For this review, take the finished solid that the model builds, in its own axes (mm). Face numbers are marked on the shaded views. A direction names the side the tool comes from. Round coordinates to 2 decimals unless told otherwise and drop trailing zeros. Order: outer loops, then holes, each group sorted by start corner. A loop starts at its lowest first (then second) coordinate and runs counter-clockwise, first axis right, second up. Notation, with made-up numbers: (26.5, -16) -> (36.5, -16) arc R21 ccw to (36.5, -11) -> close; hole circle Ø11 at (8.25, 58.5). An arc over 180 degrees is marked (long way). Answer in a Markdown table with one row per item.
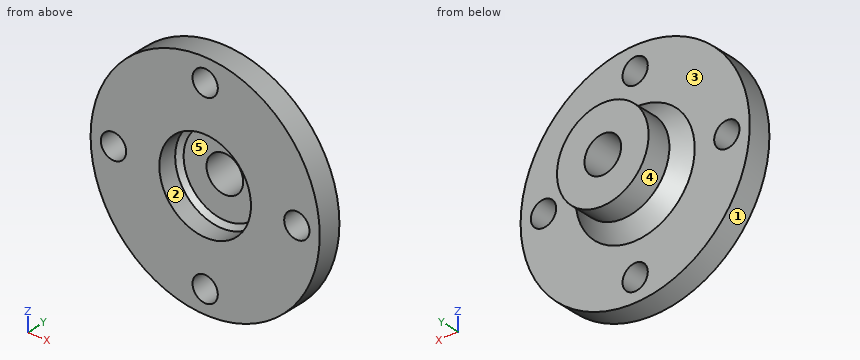
Autodesk Inventor part; units mm, degrees
ref_plane "Work Plane3" through (0, 8.5344, 0) normal (1, 0, 0) x (0, 1, 0)
ref_plane "YZ Plane" through (0, 0, 0) normal (1, 0, 0) x (0, 1, 0)
ref_plane "XZ Plane" through (0, 0, 0) normal (0, 1, 0) x (-1, 0, 0)
sketch "Sketch1" plane through (0, 0, 0) normal (0, 1, 0) x (-1, 0, 0)
  circle A0 centre (0, 0) radius 15.875
  circle A1 centre (0, 0) radius 6.35
  circle A2 centre (0, 12.7) radius 1.75
  circle A3 centre (-12.7, 0) radius 1.75
  circle A4 centre (0, -12.7) radius 1.75
  circle A5 centre (12.7, 0) radius 1.75
  dimension "d1" = 12.7
  dimension "d6" = 3.5
  dimension "d7" = 3.5
  dimension "d8" = 3.5
  dimension "d9" = 3.5
extrude "Extrusion1" add sketch "Sketch1" along normal blind 3.2258
sketch "Sketch2" plane through (0, 3.2258, 0) normal (0, 1, 0) x (1, 0, 0)
  circle A0 centre (0, 0) radius 6.35
  circle A1 centre (0, 0) radius 2.54
  dimension "d12" = 5.08
extrude "Extrusion2" add sketch "Sketch2" along normal blind 5.3086
sketch "Sketch3" plane through (0, 8.5344, 0) normal (0, 1, 0) x (1, 0, 0)
  line L0 (0, 0) -> (6.35, 0)
  circle A0 centre (0, 0) radius 6.35
  line L1 (0, 0) -> (-6.35, 0)
ref_plane "Work Plane3" through (0, 8.5344, 0) normal (1, 0, 0) x (0, 1, 0)
sketch "Sketch5" plane through (0, 3.2258, 0) normal (0, 1, 0) x (1, 0, 0)
  circle A0 centre (0, 0) radius 6.35
  circle A1 centre (0, 0) radius 8.255
  dimension "d17" = 16.51
extrude "Extrusion3" add sketch "Sketch5" along normal blind 1.905
chamfer "Chamfer1" distance 1.905 angle 45 1 edges at (-8.255, 5.1308, 0)
chamfer "Chamfer2" distance 0.635 angle 45 1 edges at (6.35, 3.2258, 0)
properties part number "FlywheelMount"
Q1. Tool access review of the marked faces 1 and 2: name each direction out of +Z, -Z, +X, -X, +Y, -Y from which nothing blocks a thin tool from reaching the whole face with its end or side.
Answer key:
| item | result |
|---|---|
| face 1 | +Y, -Y |
| face 2 | -Y |
Q2. Take a section at A-A, the plane z = 0. Give the number of separate pieces and of enclosed holes in the cut face, then the cut area to 3 significant figures.
Answer key:
| item | result |
|---|---|
| separate pieces | 4 |
| enclosed holes | 0 |
| area | 83.4 mm^2 |
Q3. The part is to be moulded in two halves that separate along X. For the marked faces 3, 4 and 5, say which applies: +X half, -X half, draft (parallel to the pull), parting line (faces both ways), or undercut.
Answer key:
| item | result |
|---|---|
| face 3 | draft |
| face 4 | parting line |
| face 5 | undercut |
Q4. Take a section at C-C, the plane x = -12.7. Write out the cut boundary in (y, z) (3 decimals).
Answer key:
| item | result |
|---|---|
| outline | (0, -9.525) -> (3.226, -9.525) -> (3.226, -1.75) -> (0, -1.75) -> close; (0, 1.75) -> (3.226, 1.75) -> (3.226, 9.525) -> (0, 9.525) -> close |
Q5. To check wall thickness, follow probe 1 along Z at (x, y) = (0, 0.6) (3 decimals); probe 2 along Z at (x, y) = (0, 6.45); probe 3 along Y at (x, z) = (-9.5, -3.5). State the ranges of each line that lie inside material, in increasing order.
Answer key:
| item | result |
|---|---|
| probe 1 | z = -15.875 to -14.45, -10.95 to -6.35, 6.35 to 10.95, 14.45 to 15.875 |
| probe 2 | z = -6.35 to -2.54, 2.54 to 6.35 |
| probe 3 | y = 0 to 3.23 |
Q6. Clearance check with flat-ended pins moving along their axes: pin 1 Ø10 at (x, z) = (0, 0) entering from +Y; pin 2 Ø5 at (x, y) = (-2, 6.5) entering from -Z; pin 3 Ø3 at (x, z) = (-12.7, 0) entering from +Y; pin 4 Ø1 at (x, y) = (9.5, 3.5) entering from +Z. State where each tip first meets the part, or that it passes through.
Answer key:
| item | result |
|---|---|
| pin 1 | stops at y = 8.53 |
| pin 2 | stops at z = -7.28 |
| pin 3 | passes through |
| pin 4 | stops at z = 13.02 |
Q7. Take a section at D-D, the plane y = 7.75. Write out the cut boundary in (x, z), then the cut area to 3 significant figures.
Answer key:
| item | result |
|---|---|
| outline | circle Ø12.7 at (0, 0); hole circle Ø5.08 at (0, 0) |
| area | 106 mm^2 |
